Could you check a few things on this drawing? It's one solid part, dimensions in mm from its lowest x, y, z. Round coordinates to 2 decimals unless told otherwise and drop trailing zeros. Loops run counter-clockwise (first coordinate to the right, second up) from the corner with the lowest first, then second, coordinate; pieces in that order, holes last. Notation, with made-up numbers: M -20.75,31 L 7.25,31 A27 ccw 7.25,61 Z; hole C 86.5,-31 d6. An arc over 180 degrees is marked long. Return JSON: item names as keys, results as strings.
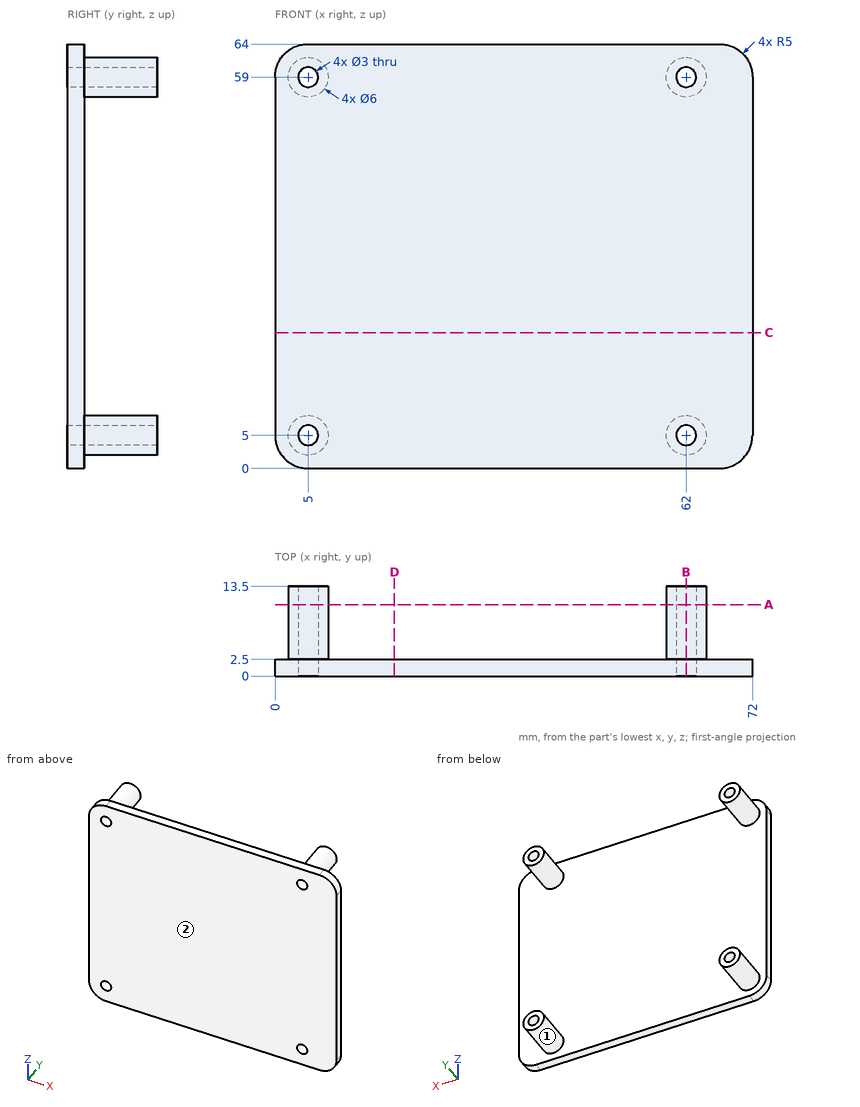
Q1. Suppose I cut it at D-D, the plane x = 18. Please give me the cut outline in (y, z).
Results:
{"outline": "M 0,0 L 2.5,0 L 2.5,64 L 0,64 Z"}
Q2. Thinking about a two-plate mould opening in X: for the marked faces 1 and 2, which applies, pulls with the +X half, pulls with the -X half, needs draft (parallel to the pull), parting line crosses it, or undercut?
Results:
{"face 1": "undercut", "face 2": "needs draft"}
Q3. Suppose I cut it at C-C, the plane z = 20.5. Please give me the cut outline in (x, y), plus the area to 3 significant figures.
Results:
{"outline": "M 0,0 L 72,0 L 72,2.5 L 0,2.5 Z", "area": "180 mm2"}
Q4. I'm going to push flat-ended pins straight in: pin 1 Ø2 at (x, z) = (26, 46.5) entering from +Y; pin 2 Ø5 at (x, y) = (58, 7.5) entering from +Z; pin 3 Ø1 at (y, z) = (8, 6.5) entering from -X. Where does each tip first touch, or does it pass through?
Results:
{"pin 1": "stops at y = 2.5", "pin 2": "stops at z = 61.6", "pin 3": "stops at x = 2.17"}
Q5. Suppose I cut it at A-A, the plane y = 10.75. Please give me the cut outline in (x, z), plus the area to 3 significant figures.
Results:
{"outline": "C 5,5 d6; C 5,59 d6; C 62,5 d6; C 62,59 d6; hole C 5,5 d3; hole C 5,59 d3; hole C 62,5 d3; hole C 62,59 d3", "area": "84.8 mm2"}
Q6. If I drill on line 1 along X through (y, z) = (7, 5); line 2 along Z through (x, y) = (4, 12.25); line 3 along Y through (x, z) = (17, 8), over which ranges is the centre line in solid material (lowest first)?
Results:
{"line 1": "x = 2 to 3.5, 6.5 to 8, 59 to 60.5, 63.5 to 65", "line 2": "z = 2.17 to 3.88, 6.12 to 7.83, 56.17 to 57.88, 60.12 to 61.83", "line 3": "y = 0 to 2.5"}
Q7. Suppose I cut it at B-B, the plane x = 62. Please give me the cut outline in (y, z).
Results:
{"outline": "M 0,0 L 2.5,0 L 2.5,2 L 13.5,2 L 13.5,3.5 L 0,3.5 Z; M 0,6.5 L 13.5,6.5 L 13.5,8 L 2.5,8 L 2.5,56 L 13.5,56 L 13.5,57.5 L 0,57.5 Z; M 0,60.5 L 13.5,60.5 L 13.5,62 L 2.5,62 L 2.5,64 L 0,64 Z"}
